For this review, take the finished solid that the model builds, in its own axes (mm). A direction names the side the tool comes from. Round coordinates to 2 decimals unless told otherwise and drop trailing zeros. Loops run counter-clockwise (first coordinate to the right, second up) from the corner with the lowest first, then second, coordinate; pieces in that order, holes last.
```python
from build123d import *

# Parameters (mm, degrees)
F4_DEPTH = 12.7
F5_DEPTH = 12.7
F2_R     = 6.35
F6_DEPTH = 8.255
F3_R     = 1.5875
F7_DEPTH = 9.525
F9_DEPTH = 5.08


with BuildPart() as f4:
    # F0 (on Front) → F4 (new body)
    with BuildSketch(Plane.XZ):
        with BuildLine():
            ThreePointArc((71.842049, 0), (43.994091, 36.817039), (0, 50.8))
            ThreePointArc((0, 50.8), (-43.994091, 36.817039), (-71.842049, 0))
            Line((-71.842049, 0), (-71.842049, -28.526883))
            ThreePointArc((-71.842049, -28.526883), (-37.607751, -45.103986), (0, -50.8))
            ThreePointArc((0, -50.8), (37.607751, -45.103986), (71.842049, -28.526883))
            Line((71.842049, -28.526883), (71.842049, 0))
        make_face()
    extrude(amount=F4_DEPTH)

    # F1 (on Front) → F5 (cut, symmetric)
    with BuildSketch(Plane.XZ):
        with BuildLine():
            ThreePointArc((62.535292, -14.373341), (40.817013, 23.243822), (0, 38.1))
            ThreePointArc((0, 38.1), (-40.817013, 23.243822), (-62.535292, -14.373341))
            Line((-62.535292, -14.373341), (-12.507058, -23.194668))
            ThreePointArc((-12.507058, -23.194668), (0, -12.7), (12.507058, -23.194668))
            Line((12.507058, -23.194668), (62.535292, -14.373341))
        make_face()
    extrude(amount=F5_DEPTH, both=True, mode=Mode.SUBTRACT)

    # F2 (on Front) → F6 (cut)
    with BuildSketch(Plane.XZ):
        with Locations((0, -25.4)):
            Circle(F2_R)
    extrude(amount=F6_DEPTH, mode=Mode.SUBTRACT)

    # F3 (on Front) → F7 (cut)
    with BuildSketch(Plane.XZ):
        with Locations((7.14464, -21.27504)):
            Circle(F3_R)
        with Locations((-16.671561, -35.02533)):
            Circle(F3_R)
    extrude(amount=F7_DEPTH, mode=Mode.SUBTRACT)

    # F8 (on face) → F9 (cut)
    with BuildSketch(Plane(origin=(0, 0, 0), x_dir=(-1, 0, 0), z_dir=(0, 1, 0))):
        Polygon((-1.96021, -16.935924), (-8.31021, -27.934446), (11.487131, -39.364446), (17.837131, -28.365924), align=None)
    extrude(amount=-F9_DEPTH, mode=Mode.SUBTRACT)


solid = f4.part
```
(1) The part is to be moulded in two halves that separate along X. For faces 4 (the flat face through (7.276, -2.504, -26.144)), 5 (the flat face through (-71.842, -6, -14)), 6 (the flat face through (71.842, -6, -14)), say which applies: pulls with the +X half, pulls with the -X half, needs draft (parallel to the pull), parting line crosses it, or undercut.
(2) For faces 1 (the flat face through (-1, -12.7, -22)), 2 (the cylindrical face through (-0.2, -6.4, -12.7)), 3 (the flat face through (-10, -5.08, -32)), list the 3-axis set-ups (+Z, -Z, +X, -X, +Y, -Y) from which the entire face can be reached by the end or side of a thin tool; tool diameter is ignored.
(3) For L1, parallel to X at y = -2.75, z = -14; L2, parallel to X at y = -4.5, z = 18.5; L3, parallel to Z at x = 41.5, y = -11, list the stretches that pass through material, from the lowest coordinate up.
(4) Add section D-D (z = 41). Give the boundary of the cut face in (x, y), plus the area to 3 significant figures.
(5) Insertion check: pin 1 Ø2 at (x, y) = (6, -4.5) entering from -Z; pin 2 Ø5 at (x, y) = (11.5, -11) entering from +Z; pin 3 Ø4 at (x, y) = (37.5, -6.5) entering from +Z. Each pin has a flat end and moves straight along its axis. Give the tip position at first contact, or say it passes through.
(6) Add section A-A (x = -41). Give the boundary of the cut face in (y, z).
(7) Add section B-B (y = -2.5). Give the number of separate pieces and of enclosed holes in the cut face, plus the area to 3 significant figures.
(8) Add section C-C (x = 40). Give the boundary of the cut face in (y, z), plus the area to 3 significant figures.
Outcome:
1. face 4: undercut
1. face 5: pulls with the -X half
1. face 6: pulls with the +X half
2. face 1: +Z, -Z, +X, -X, -Y
2. face 2: +Y, -Y
2. face 3: +Y
3. L1: x = -71.84 to -62.47, -5.6 to 5.6, 62.47 to 71.84
3. L2: x = -62.28 to -45.88, 45.88 to 62.28
3. L3: z = -43.83 to -18.08, 22.66 to 38.51
4. outline: (-37.38, -12.7) - (37.38, -12.7) - (37.38, 0) - (-37.38, 0) - close
4. area: 950 mm2
5. pin 1: stops at z = -50.7
5. pin 2: stops at z = 50.27
5. pin 3: stops at z = 42.03
6. outline: (-12.7, -44) - (0, -44) - (0, -18.17) - (-12.7, -18.17) - close; (-12.7, 23.09) - (0, 23.09) - (0, 38.83) - (-12.7, 38.83) - close
7. separate pieces: 1
7. enclosed holes: 4
7. area: 5,880 mm2
8. outline: (-12.7, -44.34) - (0, -44.34) - (0, -18.35) - (-12.7, -18.35) - close; (-12.7, 23.92) - (0, 23.92) - (0, 39.46) - (-12.7, 39.46) - close
8. area: 527 mm2
